Check sheet for the modelled part. Datum: model origin and axes. Units: mm. Round coordinates to 2 decimals unless told otherwise and drop trailing zeros. Loops run counter-clockwise (first coordinate to the right, second up) from the corner with the lowest first, then second, coordinate; pieces in that order, holes last. Notation, with made-up numbers: (69.5, -32) -> (88.5, -32) arc R12 cw to (88.5, -10) -> close; hole circle Ø7 at (86.5, 19.5). An arc over 180 degrees is marked (long way). Return JSON: item names as keys, results as strings.
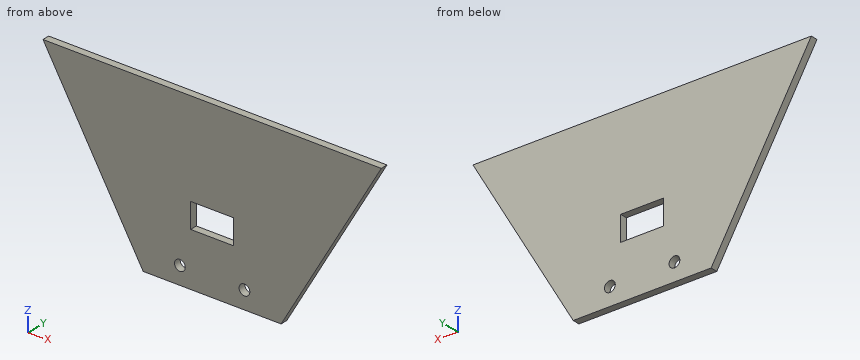
from build123d import *

# Parameters (mm, degrees)
ESQUISSE1_R        = 1.5
ESQUISSE1_W        = 12
ESQUISSE1_H        = 7
BOSS_EXTRU_1_DEPTH = 2


with BuildPart() as part:
    # Esquisse1 → Boss.-Extru.1 (new body)
    with BuildSketch(Plane(origin=(0, 0, 0), x_dir=(1, 0, 0), z_dir=(0, 1, 0))):
        Polygon((-18.31712618, 39.132721947), (20.135868436, 39.132721947), (48.074434638, -9.258294204), (-46.255692381, -9.258294204), align=None)
        with Locations((-8.090628872, 34.132721947)):
            Circle(ESQUISSE1_R, mode=Mode.SUBTRACT)
        with Locations((9.909371128, 34.132721947)):
            Circle(ESQUISSE1_R, mode=Mode.SUBTRACT)
        with Locations((0.909371128, 20.632721947)):
            Rectangle(ESQUISSE1_W, ESQUISSE1_H, mode=Mode.SUBTRACT)
    extrude(amount=BOSS_EXTRU_1_DEPTH)


solid = part.part
Q1. Section check B-B (z = -19). Record the boundary of the cut face in (x, y), then the cut area to 3 significant figures.
Results list:
{"outline": "(-29.94, 0) -> (-5.09, 0) -> (-5.09, 2) -> (-29.94, 2) -> close; (6.91, 0) -> (31.76, 0) -> (31.76, 2) -> (6.91, 2) -> close", "area": "99.4 mm^2"}
Q2. Go/stop test with flat-tipped pins: pin 1 (0.6 mm diameter, centred on y = 1, z = -21.5, fed in from -X); pin 2 (1 mm diameter, centred on y = 0.5, z = -16, fed in from -X); pin 3 (10 mm diameter, centred on x = 1, z = -22, fed in from +Y); pin 4 (0.6 mm diameter, centred on y = 1, z = -21, fed in from +X). Record where each tip stops, or that it passes through.
Results list:
{"pin 1": "x = -28.67", "pin 2": "x = -31.96", "pin 3": "y = 2", "pin 4": "x = 30.78"}
Q3. Section check C-C (y = 0.8). Record the boundary of the cut face in (x, z).
Results list:
{"outline": "(-46.26, 9.26) -> (-18.32, -39.13) -> (20.14, -39.13) -> (48.07, 9.26) -> close; hole circle Ø3 at (-8.09, -34.13); hole (-5.09, -24.13) -> (6.91, -24.13) -> (6.91, -17.13) -> (-5.09, -17.13) -> close; hole circle Ø3 at (9.91, -34.13)"}
Q4. Section check D-D (z = -2). Record the boundary of the cut face in (x, y).
Results list:
{"outline": "(-39.76, 0) -> (41.57, 0) -> (41.57, 2) -> (-39.76, 2) -> close"}
Q5. Material ranges on line 1 (Z direction, x = -2.5, y = 0.85); line 2 (X direction, y = 1, z = -33.5); line 3 (X direction, y = 1.7, z = -23), recorded low to high.
Results list:
{"line 1": "-39.13 to -24.13, -17.13 to 9.26", "line 2": "-21.57 to -9.45, -6.73 to 8.55, 11.27 to 23.39", "line 3": "-27.63 to -5.09, 6.91 to 29.45"}
Q6. Section check A-A (x = 3.5). Record the boundary of the cut face in (y, z), then the cut area to 3 significant figures.
Results list:
{"outline": "(0, -39.13) -> (2, -39.13) -> (2, -24.13) -> (0, -24.13) -> close; (0, -17.13) -> (2, -17.13) -> (2, 9.26) -> (0, 9.26) -> close", "area": "82.8 mm^2"}
